Here's how the part is built. I have some questions about the finished solid (model axes, mm). Face numbers are marked on the shaded views. A direction names the side the tool comes from. Round coordinates to 2 decimals unless told otherwise and drop trailing zeros. Order: outer loops, then holes, each group sorted by start corner. A loop starts at its lowest first (then second) coordinate and runs counter-clockwise, first axis right, second up. Notation, with made-up numbers: M -18,36 L -8,36 A36 ccw -8,75 Z; hole C -31.5,74 d4. An arc over 180 degrees is marked long. Write item = value, one per line. Start each with the question number.
Item 1: I want a section at C-C, the plane x = 4. List the corners of the cut face in (y, z) for me.
Item 2: Please list where these lines run through material, in increasing order: L1, parallel to Y at x = 3, z = -1; L2, parallel to Y at x = 21.5, z = 0; L3, parallel to Z at x = 22, y = -1.5.
Item 3: I'm going to push flat-ended pins straight in: P1, Ø3.5, axis at x = 1, z = -1, coming from the -Y side (3 decimals); P2, Ø4, axis at x = 21, y = -4.5, coming from the +Z side; P3, Ø2, axis at x = 3, z = -0.5, coming from the +Y side; P4, Ø3.5, axis at x = 2.5, y = 0, coming from the -Z side. Where does each tip first touch, or does it pass through?
Item 4: I want a section at A-A, the plane z = 0. List the corners of the cut face in (x, y) for me (3 decimals).
Item 5: I want a section at D-D, the plane x = 16.5. List the corners of the cut face in (y, z) for me, plus the area to 3 significant figures.
Item 6: For the marked faces 1, 2, 3 and 4, which set-ups out of +Z, -Z, +X, -X, +Y, -Y let a thin tool reach every point of the face, with its end or its side?
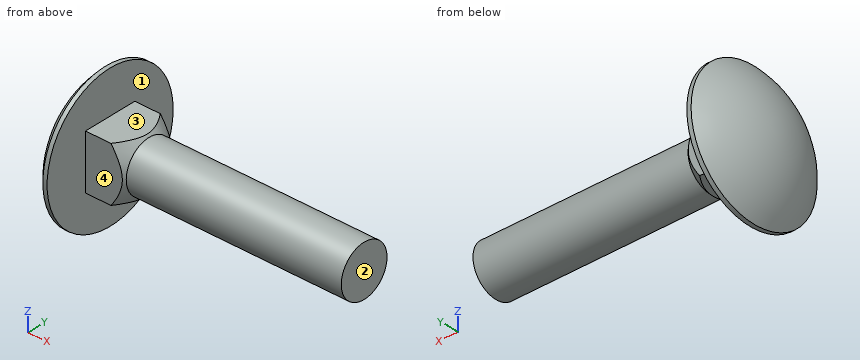
```python
from build123d import *

# Parameters (mm, degrees)
SKETCH_2_W      = 6.48
SKETCH_2_H      = 6.48
EXTRUDE_1_DEPTH = 4.6


with BuildPart() as part:
    # Эскиз1 → Повернуть1 (revolve)
    with BuildSketch(Plane.XY):
        with BuildLine():
            Line((30, 0), (-3.88, 0))
            ThreePointArc((-3.88, 0), (-3.002420637, 4.469340695), (-0.5, 8.275))
            Line((-0.5, 8.275), (0, 8.275))
            Line((0, 8.275), (0, 3))
            Line((0, 3), (30, 3))
            Line((30, 3), (30, 0))
        make_face()
    revolve(axis=Axis((-946.390579576, 0, 0), (1, 0, 0)))

    # Эскиз2 → Бобышка-Вытянуть1 (add)
    with BuildSketch(Plane(origin=(0, 0, 0), x_dir=(0, 0, -1), z_dir=(1, 0, 0))):
        Rectangle(SKETCH_2_W, SKETCH_2_H)
    extrude(amount=EXTRUDE_1_DEPTH)


with BuildPart() as body_2:
    # Эскиз3 → Повернуть2 (revolve)
    with BuildSketch(Plane(origin=(0, 0, 0), x_dir=(-1, 0, 0), z_dir=(0, -0.707106781, 0.707106781))):
        Polygon((-4.6, 3), (-2.017948058, 5.582051942), (-7.182051942, 5.582051942), align=None)
    revolve(axis=Axis((1000, 0, 0), (-1, 0, 0)))


with BuildPart() as part_1:
    add(part.part)

    # Combine 1: cut body 2
    add(body_2.part, mode=Mode.SUBTRACT)


solid = part_1.part
```
Filled in:
q1.outline = M -3.24,-1.57 A3.6 ccw -1.57,-3.24 L 1.57,-3.24 A3.6 ccw 3.24,-1.57 L 3.24,1.57 A3.6 ccw 1.57,3.24 L -1.57,3.24 A3.6 ccw -3.24,1.57 Z
q2.L1 = -3.24 to 3.24
q2.L2 = -3 to 3
q2.L3 = -2.6 to 2.6
q3.P1 = -8.275
q3.P2 = 1.66
q3.P3 = 3.24
q3.P4 = -3.24
q4.outline = M -0.5,-8.275 L 0,-8.275 L 0,-3.24 L 4.36,-3.24 L 4.6,-3 L 30,-3 L 30,3 L 4.6,3 L 4.36,3.24 L 0,3.24 L 0,8.275 L -0.5,8.275 A11.82 ccw Z
q5.outline = C 0,0 d6
q5.area = 28.3 mm^2
q6.face_1 = +X
q6.face_2 = +Z, -Z, +X, +Y, -Y
q6.face_3 = +Z, +X, +Y, -Y
q6.face_4 = +Z, -Z, +X, -Y
